Input: part model. Units: mm. Frame: model coordinates. A direction names the side the tool comes from. Give positions to 0.01 mm unless a question says otherwise; leave off trailing zeros. Loops run counter-clockwise (first coordinate to the right, second up) from the corner with the lowest first, then second, coordinate; pieces in that order, holes last. Notation, with made-up numbers: M 17.25,-8.5 L 61.25,-8.5 A4 cw 61.25,-2.5 Z; hole C 23,-31.75 d8. An arc over 180 degrees is marked long. One line per item, written item: value. Start each with the question number.
(1) Section C-C on z = -11. Output: boundary loops of the cut face in (x, y), plus the area to 3 significant figures.
(2) Section D-D on y = 10. Output: boundary loops of the cut face in (x, z), plus the area to 3 significant figures.
(3) Pin query (flat end, axial travel): P1, Ø12, axis at y = 26.5, z = 13, coming from the -X side; P2, Ø23, axis at x = 0, z = 0, coming from the -Y side; P3, Ø2, axis at y = 29.5, z = 0.5, coming from the +X side; P4, Ø2.5, axis at y = 10, z = 0, coming from the -X side. Return the tip coordinate at first contact, or that it passes through.
(4) Section A-A on z = 0. Output: boundary loops of the cut face in (x, y), plus the area to 3 significant figures.
(5) Pull-direction query (Z, two-part tool) for faces 1 (the cylindrical face through (-22.2, 48.3, 11.5)), 2 (the flat face through (26, 40, -2)), 3 (the flat face through (20, 10, 0)), 4 (the cylindrical face through (25.07, 11.897, -1.21)); classes: released by +Z, released by -Z, zero draft, split by the parting line, or undercut.
(6) Ray query, line 1 along Y through (x, z) = (24.25, 0); line 2 along Y through (x, z) = (25.5, 0); line 3 along Z through (x, y) = (-0.5, 60) (3 decimals). Return the intervals inside material, ascending. Write a range as from..to.
(7) Access query for faces 5 (the cylindrical face through (-18.75, 11.18, -0.75)), 6 (the flat face through (20, 30, 0)), 7 (the flat face through (30, 20, 0)). Directions: +Z, -Z, +X, -X, +Y, -Y. A direction counts if a zero-diameter tool reaches every point of the face in a straight line with its end or side. Return the directions, or none.
(8) Section B-B on x = 8. Output: boundary loops of the cut face in (y, z).
```python
from build123d import *

# Parameters (mm, degrees)
SKETCH1_R                       = 25
BOSS_EXTRUDE1_DEPTH             = 80
SKETCH2_R                       = 12.75
CUT_EXTRUDE1_DEPTH              = 88.464278423
SKETCH3_R                       = 1.4
CUT_EXTRUDE2_DEPTH              = 88.464278423
BOSS_EXTRUDE2_REACH             = 99.596
BOSS_EXTRUDE2_END_RADIUS        = 25
SKETCH5_W                       = 50
SKETCH5_H                       = 40
BOSS_EXTRUDE2_DIRECTION_2_DEPTH = 5
SKETCH6_R                       = 2.25
CUT_EXTRUDE3_DEPTH              = 10


with BuildPart() as part:
    # Sketch1 → Boss-Extrude1 (new body)
    with BuildSketch(Plane(origin=(0, 0, 0), x_dir=(1, 0, 0), z_dir=(0, 1, 0))):
        with Locations(Location((0, 0, 0), (0, 0, 270))):
            Circle(SKETCH1_R)
    extrude(amount=BOSS_EXTRUDE1_DEPTH)

    # Sketch2 → Cut-Extrude1 (cut, through all)
    with BuildSketch(Plane(origin=(0, 80, 0), x_dir=(1, 0, 0), z_dir=(0, 1, 0))):
        with Locations(Location((0, 0, 0), (0, 0, 270))):
            Circle(SKETCH2_R)
    extrude(amount=-CUT_EXTRUDE1_DEPTH, mode=Mode.SUBTRACT)

    # Sketch3 → Cut-Extrude2 (cut, through all)
    with BuildSketch(Plane(origin=(0, 0, 0), x_dir=(0, 0, -1), z_dir=(1, 0, 0))):
        with Locations((0, 30)):
            Circle(SKETCH3_R)
        with Locations((0, 10)):
            Circle(SKETCH3_R)
    extrude(amount=-CUT_EXTRUDE2_DEPTH, mode=Mode.SUBTRACT)

    # Boss-Extrude2: up to this cylinder (the profile starts outside it)
    boss_extrude2_end = Plane(origin=(0, 20, 0), z_dir=(0, -1, 0)) * Cylinder(BOSS_EXTRUDE2_END_RADIUS, 250.192, mode=Mode.PRIVATE)
    # Sketch5 → Boss-Extrude2 (add, up to the surface)
    with BuildSketch(Plane(origin=(25, 0, 0), x_dir=(0, 0, -1), z_dir=(1, 0, 0)), mode=Mode.PRIVATE) as boss_extrude2_sk1:
        with Locations((0, 20)):
            Rectangle(SKETCH5_W, SKETCH5_H)
    boss_extrude2_tool1 = extrude(boss_extrude2_sk1.sketch, amount=-BOSS_EXTRUDE2_REACH, mode=Mode.PRIVATE) - boss_extrude2_end
    add(boss_extrude2_tool1.solids().sort_by_distance((25, 20, 0))[0])
    add(boss_extrude2_tool1.solids().sort_by_distance((25, 20, 0))[1])

    # Sketch5 → Boss-Extrude2 direction 2 (add)
    with BuildSketch(Plane(origin=(25, 0, 0), x_dir=(0, 0, -1), z_dir=(1, 0, 0))):
        with Locations((0, 20)):
            Rectangle(SKETCH5_W, SKETCH5_H)
    extrude(amount=BOSS_EXTRUDE2_DIRECTION_2_DEPTH)

    # Sketch6 → Cut-Extrude3 (cut)
    with BuildSketch(Plane(origin=(30, 0, 0), x_dir=(0, 0, -1), z_dir=(1, 0, 0))):
        with Locations((0, 10)):
            Circle(SKETCH6_R)
        with Locations((0, 30)):
            Circle(SKETCH6_R)
    extrude(amount=-CUT_EXTRUDE3_DEPTH, mode=Mode.SUBTRACT)


solid = part.part
```
Output values:
1. outline: M -22.45,0 L -6.45,0 L -6.45,80 L -22.45,80 Z; M 6.45,0 L 30,0 L 30,40 L 22.45,40 L 22.45,80 L 6.45,80 Z
1. area: 2,860 mm²
2. outline: M -24.96,-1.4 A25 ccw 0,-25 L 30,-25 L 30,-2.25 L 20,-2.25 L 20,2.25 L 30,2.25 L 30,25 L 0,25 A25 ccw -24.96,1.4 L -12.67,1.4 A12.75 cw long -12.67,-1.4 Z
2. area: 1,890 mm²
3. P1: stops at x = -24
3. P2: passes through
3. P3: stops at x = 20
3. P4: stops at x = 12.69
4. outline: M -25,0 L -12.75,0 L -12.75,8.6 L -25,8.6 Z; M -25,11.4 L -12.75,11.4 L -12.75,28.6 L -25,28.6 Z; M -25,31.4 L -12.75,31.4 L -12.75,80 L -25,80 Z; M 12.75,0 L 30,0 L 30,7.75 L 20,7.75 L 20,12.25 L 30,12.25 L 30,27.75 L 20,27.75 L 20,32.25 L 30,32.25 L 30,40 L 25,40 L 25,80 L 12.75,80 Z
4. area: 2,000 mm²
5. face 1: split by the parting line
5. face 2: zero draft
5. face 3: undercut
5. face 4: undercut
6. line 1: y = 0..7.75, 12.25..27.75, 32.25..80
6. line 2: y = 0..7.75, 12.25..27.75, 32.25..40
6. line 3: z = -24.995..-12.74, 12.74..24.995
7. face 5: -X
7. face 6: +X
7. face 7: +Z, -Z, +X, +Y, -Y
8. outline: M 0,-25 L 40,-25 L 40,-23.69 L 80,-23.69 L 80,-9.93 L 0,-9.93 Z; M 0,9.93 L 80,9.93 L 80,23.69 L 40,23.69 L 40,25 L 0,25 Z
